Input: part model. Units: mm. Frame: model coordinates. Face numbers are marked on the shaded views. Round coordinates to 2 decimals unless told otherwise and drop trailing zeros. Write each loop counter-clockwise with the first axis right and the second up, starting at its lowest first coordinate (ties: lowest second). Pieces come first, ordered by that corner, then holes. Notation, with made-up numbers: (62.25, 67.5) -> (92.25, 67.5) arc R12 ccw to (92.25, 86.5) -> close; hole circle Ø8 at (36.25, 24). An arc over 180 degrees is marked (long way). Write item = value, one per line. Start each with the question number.
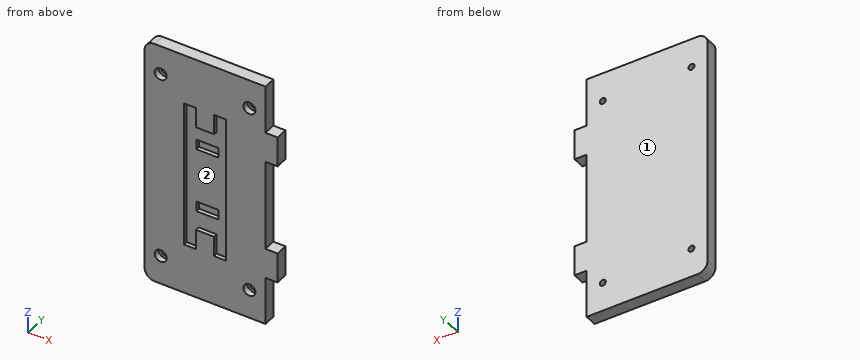
```python
from build123d import *

# Parameters (mm, degrees)
BOSS_EXTRU_1_DEPTH      = 6
ESQUISSE3_R             = 1.5
ENL_V_MAT_EXTRU_1_DEPTH = 6
CONG_1_R                = 5
ESQUISSE6_R             = 3
ENL_V_MAT_EXTRU_2_DEPTH = 3
ENL_V_MAT_EXTRU_3_DEPTH = 2
ESQUISSE8_W             = 11
ESQUISSE8_H             = 5
ENL_V_MAT_EXTRU_4_DEPTH = 2


with BuildPart() as part:
    # Esquisse1 → Boss.-Extru.1 (new body)
    with BuildSketch(Plane(origin=(0, 0, 0), x_dir=(1, 0, 0), z_dir=(0, 1, 0))):
        Polygon((-30, 61.38), (30, 61.38), (30, 37.5), (36, 37.5), (36, 22.5), (30, 22.5), (30, -22.5), (36, -22.5), (36, -37.5), (30, -37.5), (30, -61.38), (-30, -61.38), align=None)
    extrude(amount=BOSS_EXTRU_1_DEPTH)

    # Esquisse3 → Enlèv. mat.-Extru.1 (cut)
    with BuildSketch(Plane(origin=(0, 6, 0), x_dir=(1, 0, 0), z_dir=(0, 1, 0))):
        with Locations(Location((22, 47, 0), (0, 0, 270))):
            Circle(ESQUISSE3_R)
        with Locations(Location((-22, 47, 0), (0, 0, 270))):
            Circle(ESQUISSE3_R)
        with Locations(Location((-22, -47, 0), (0, 0, 90))):
            Circle(ESQUISSE3_R)
        with Locations(Location((22, -47, 0), (0, 0, 90))):
            Circle(ESQUISSE3_R)
    extrude(amount=-ENL_V_MAT_EXTRU_1_DEPTH, mode=Mode.SUBTRACT)

    # Congé1
    cong_1_edges = [part.edges().sort_by_distance(p)[0] for p in [
        (-30, 3, -61.38),
        (-30, 3, 61.38),
    ]]
    fillet(cong_1_edges, radius=CONG_1_R)

    # Esquisse6 → Enlèv. mat.-Extru.2 (cut)
    with BuildSketch(Plane.XZ):
        with Locations(Location((22, 47, 0), (0, 0, 270))):
            Circle(ESQUISSE6_R)
        with Locations(Location((-22, 47, 0), (0, 0, 270))):
            Circle(ESQUISSE6_R)
        with Locations(Location((22, -47, 0), (0, 0, 270))):
            Circle(ESQUISSE6_R)
        with Locations(Location((-22, -47, 0), (0, 0, 270))):
            Circle(ESQUISSE6_R)
    extrude(amount=-ENL_V_MAT_EXTRU_2_DEPTH, mode=Mode.SUBTRACT)

    # Esquisse7 → Enlèv. mat.-Extru.3 (cut)
    with BuildSketch(Plane(origin=(0, 0, 0), x_dir=(-1, 0, 0), z_dir=(0, -1, 0))):
        Polygon((10.5, -36.5), (10.5, 36.5), (4.5, 36.5), (4.5, 26.5), (-4.5, 26.5), (-4.5, 36.5), (-10.5, 36.5), (-10.5, -36.5), (-4.5, -36.5), (-4.5, -26.5), (4.5, -26.5), (4.5, -36.5), align=None)
    extrude(amount=-ENL_V_MAT_EXTRU_3_DEPTH, mode=Mode.SUBTRACT)

    # Esquisse8 → Enlèv. mat.-Extru.4 (cut)
    with BuildSketch(Plane(origin=(0, 2, 0), x_dir=(-1, 0, 0), z_dir=(0, -1, 0))):
        with Locations((0, -16)):
            Rectangle(ESQUISSE8_W, ESQUISSE8_H)
        with Locations((0, 16)):
            Rectangle(ESQUISSE8_W, ESQUISSE8_H)
    extrude(amount=-ENL_V_MAT_EXTRU_4_DEPTH, mode=Mode.SUBTRACT)


solid = part.part
```
1. Section D-D (x = 7). Output: boundary loops of the cut face in (y, z).
2. Section C-C (x = 22). Output: boundary loops of the cut face in (y, z).
3. Section A-A (y = 0.9). State how many separate pieces and enclosed holes the cut face has, then the cut area to 3 significant figures.
4. Pin query (flat end, axial travel): P1, Ø4, axis at x = -2.5, z = 2, coming from the -Y side; P2, Ø1.5, axis at x = 2, z = -15, coming from the -Y side; P3, Ø1.8, axis at x = 34, y = 4.5, coming from the +Z side. Return the tip coordinate at first contact, or that it passes through.
5. Section B-B (z = -47). Output: boundary loops of the cut face in (x, y), then the cut area to 3 significant figures.
6. Line query: line 1 along X through (y, z) = (1.15, 47); line 2 along X through (y, z) = (4.4, -47); line 3 along Z through (x, y) = (3, 3.35). Output: solid intervals per line, ascending.
7. Mould query, pull axis Z, two halves, no side actions, for the marked faces 1 and 2. Classes: pulls with the +Z half, pulls with the -Z half, needs draft (parallel to the pull), parting line crosses it, or undercut.
Check sheet entries:
q1.outline = (0, -61.38) -> (6, -61.38) -> (6, 61.38) -> (0, 61.38) -> (0, 36.5) -> (2, 36.5) -> (2, -36.5) -> (0, -36.5) -> close
q2.outline = (0, -61.38) -> (6, -61.38) -> (6, -48.5) -> (3, -48.5) -> (3, -50) -> (0, -50) -> close; (0, -44) -> (3, -44) -> (3, -45.5) -> (6, -45.5) -> (6, 45.5) -> (3, 45.5) -> (3, 44) -> (0, 44) -> close; (0, 50) -> (3, 50) -> (3, 48.5) -> (6, 48.5) -> (6, 61.38) -> (0, 61.38) -> close
q3.separate_pieces = 1
q3.enclosed_holes = 5
q3.area = 6,070 mm2
q4.P1 = 2
q4.P2 = 4
q4.P3 = 37.5
q5.outline = (-30, 0) -> (-25, 0) -> (-25, 3) -> (-23.5, 3) -> (-23.5, 6) -> (-30, 6) -> close; (-20.5, 3) -> (-19, 3) -> (-19, 0) -> (19, 0) -> (19, 3) -> (20.5, 3) -> (20.5, 6) -> (-20.5, 6) -> close; (23.5, 3) -> (25, 3) -> (25, 0) -> (30, 0) -> (30, 6) -> (23.5, 6) -> close
q5.area = 306 mm2
q6.line_1 = -30 to -25, -19 to 19, 25 to 30
q6.line_2 = -30 to -23.5, -20.5 to 20.5, 23.5 to 30
q6.line_3 = -61.38 to -18.5, -13.5 to 13.5, 18.5 to 61.38
q7.face_1 = needs draft
q7.face_2 = undercut
